from build123d import *

# Parameters (mm, degrees)
F0_R     = 20
F0_R_2   = 8
F1_DEPTH = 20
F2_R     = 10
F2_R_2   = 8
F3_DEPTH = 20
F4_R     = 4
F5_DEPTH = 25


with BuildPart() as f1:
    # F0 (on Top) → F1 (new body)
    with BuildSketch(Plane.XY):
        Circle(F0_R)
        Circle(F0_R_2, mode=Mode.SUBTRACT)
    extrude(amount=F1_DEPTH)

    # F2 (on face) → F3 (join)
    with BuildSketch(Plane(origin=(0, 0, 0), x_dir=(1, 0, 0), z_dir=(0, 0, -1))):
        Circle(F2_R)
        Circle(F2_R_2, mode=Mode.SUBTRACT)
    extrude(amount=F3_DEPTH)

    # F4 (on Front) → F5 (cut)
    with BuildSketch(Plane.XZ):
        with Locations((0, 10)):
            Circle(F4_R)
    extrude(amount=-F5_DEPTH, mode=Mode.SUBTRACT)


solid = f1.part
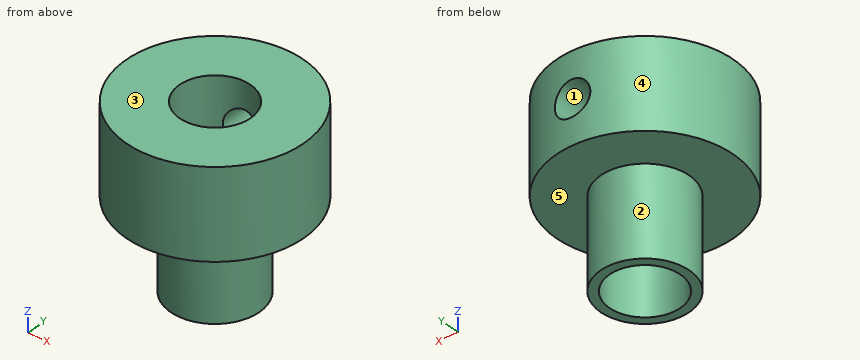
Design review of the part built by this model. Coordinates are the model's own, in mm. Face numbers are marked on the shaded views. A direction names the side the tool comes from. Round coordinates to 2 decimals unless told otherwise and drop trailing zeros. Write each loop counter-clockwise with the first axis right and the second up, starting at its lowest first coordinate (ties: lowest second). Pieces come first, ordered by that corner, then holes. Notation, with made-up numbers: (80.25, 33.25) - (86.25, 33.25) arc R12 cw to (86.25, 44.25) - close; hole circle Ø5 at (52, -29.75). An arc over 180 degrees is marked (long way). Use a Markdown table: item, result. Add a question column.
1. We need section A-A (x = 0). State the section outline as (y, z) points.
2. We need section C-C (x = -5). State the section outline as (y, z) points (3 decimals), then the cut area to 3 significant figures.
3. Clearance check with flat-ended pins moving along their axes: pin 1 (4 mm diameter, centred on y = -4, z = 12.5, fed in from +X); pin 2 (12 mm diameter, centred on x = 1, z = -8, fed in from +Y); pin 3 (4 mm diameter, centred on x = -16, z = 1, fed in from +Y). State where each tip first meets the part, or that it passes through.
4. Wall thickness on probe 1 along Z at (x, y) = (0, 16); probe 2 along Y at (x, z) = (0, -9); probe 3 along Z at (x, y) = (10, 3.5): over which ranges is each line inside the solid? List them lowest first.
5. Mouldability with a two-part tool opening along Z and no side actions: class the marked faces 1, 2 and 3 as +Z half, -Z half, draft (parallel to the pull), parting line (faces both ways), or undercut.
6. We need section B-B (y = 0). State the section outline as (x, z) points, then the cut area to 3 significant figures.
7. For the marked faces 4 and 5, list the 3-axis set-ups (+Z, -Z, +X, -X, +Y, -Y) from which the entire face can be reached by the end or side of a thin tool; tool diameter is ignored.
8. We need section D-D (z = 3.5). State the section outline as (x, y) points.
Output:
| question | item | result |
|---|---|---|
| 1 | outline | (-20, 0) - (-10, 0) - (-10, -20) - (-8, -20) - (-8, 20) - (-20, 20) - close; (8, -20) - (10, -20) - (10, 0) - (20, 0) - (20, 6) - (8, 6) - close; (8, 14) - (20, 14) - (20, 20) - (8, 20) - close |
| 2 | outline | (-19.365, 0) - (-8.66, 0) - (-8.66, -20) - (-6.245, -20) - (-6.245, 20) - (-19.365, 20) - close; (6.245, -20) - (8.66, -20) - (8.66, 0) - (19.365, 0) - (19.365, 20) - (6.245, 20) - close |
| 2 | area | 621 mm2 |
| 3 | pin 1 | stops at x = 19.9 |
| 3 | pin 2 | stops at y = 10 |
| 3 | pin 3 | stops at y = 14.28 |
| 4 | probe 1 | z = 0 to 6, 14 to 20 |
| 4 | probe 2 | y = -10 to -8, 8 to 10 |
| 4 | probe 3 | z = 0 to 20 |
| 5 | face 1 | undercut |
| 5 | face 2 | draft |
| 5 | face 3 | +Z half |
| 6 | outline | (-20, 0) - (-10, 0) - (-10, -20) - (-8, -20) - (-8, 20) - (-20, 20) - close; (8, -20) - (10, -20) - (10, 0) - (20, 0) - (20, 20) - (8, 20) - close |
| 6 | area | 560 mm2 |
| 7 | face 4 | +Z, -Z |
| 7 | face 5 | -Z |
| 8 | outline | circle Ø40 at (0, 0); hole circle Ø16 at (0, 0) |
